Answer from the drawing. Dimensions are ordinates in mm from the lowest x, y and z of the part. Round coordinates to 2 decimals unless told otherwise and drop trailing zeros. Order: outer loops, then holes, each group sorted by start corner. A loop starts at its lowest first (then second) coordinate and runs counter-clockwise, first axis right, second up. Notation, with made-up numbers: (-21.75, 23) -> (36.25, 23) arc R28 cw to (36.25, 46) -> close; hole circle Ø5 at (77, -5). An arc over 180 degrees is marked (long way). Use a Markdown table: item, result. Add a question column.
Item 1: For a pull along Z with two mould halves and no side action, classify the marked faces 1 and 2 as +Z half, -Z half, draft (parallel to the pull), parting line (faces both ways), or undercut.
Item 2: Find the intervals of material crossed by L1, parallel to X at y = 1.1, z = 78.35; L2, parallel to X at y = 2.2, z = 78.35; L3, parallel to Y at x = 28.5, z = 90.5, in increasing order. Write a range as [from, to].
Item 3: Flat-ended cylindrical pins translate along their axes: P1, Ø1.5, axis at y = 11.5, z = 92, coming from the -X side; P2, Ø2, axis at x = 66, z = 109, coming from the +Y side; P3, Ø1.5, axis at x = 98, y = 4, coming from the +Z side; P4, Ø7, axis at x = 140.85, z = 78.35, coming from the -Y side. Find the tip coordinate at first contact, or state that the pin passes through.
Item 4: A cutting plane is placed at D-D, the plane x = 15.85. Determine the outline of the cut face in (y, z).
Item 5: A cutting plane is placed at B-B, the plane x = 78.35. Determine the outline of the cut face in (y, z).
Item 6: A cutting plane is placed at A-A, the plane z = 78.35. Determine the outline of the cut face in (x, y), plus the area to 4 significant figures.
Item 7: A cutting plane is placed at C-C, the plane z = 15.85. Determine the outline of the cut face in (x, y).
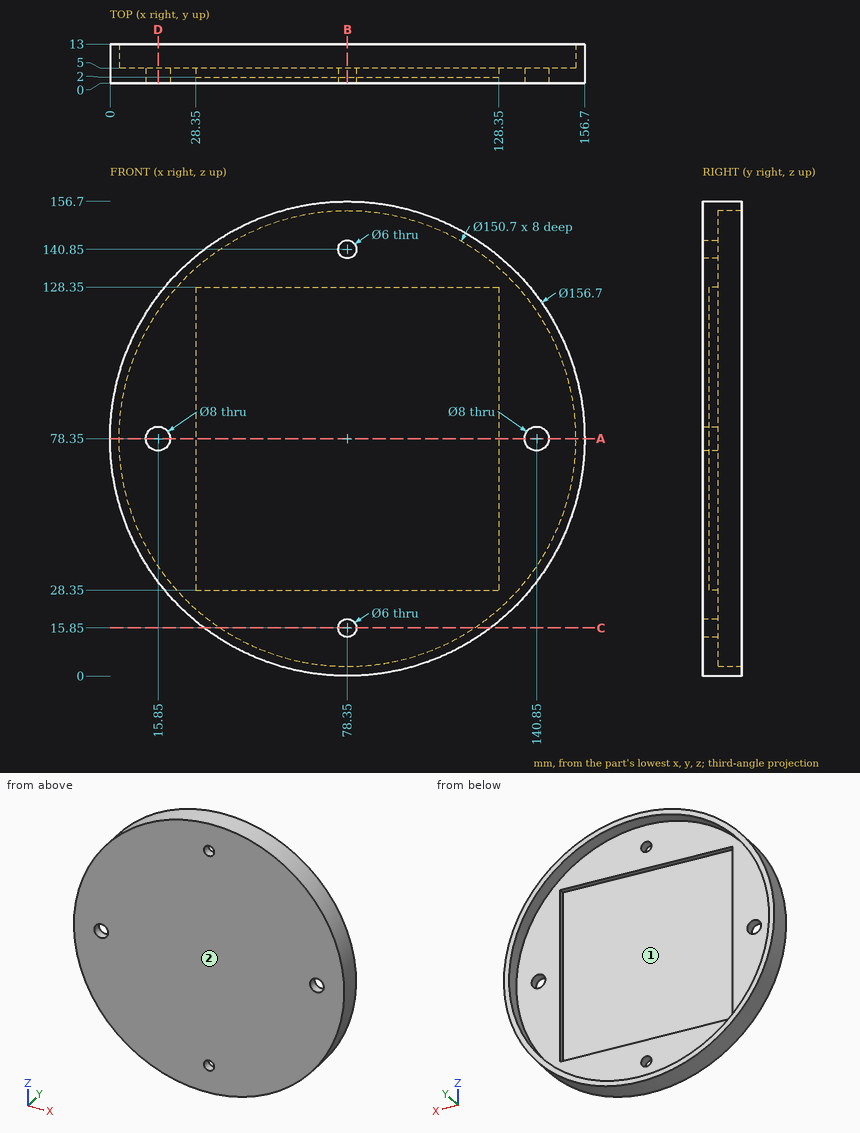
Reported:
| question | item | result |
|---|---|---|
| 1 | face 1 | undercut |
| 1 | face 2 | draft |
| 2 | L1 | [0, 11.85], [19.85, 136.85], [144.85, 156.7] |
| 2 | L2 | [0, 11.85], [19.85, 28.35], [128.35, 136.85], [144.85, 156.7] |
| 2 | L3 | [0, 2] |
| 3 | P1 | x = 1.07 |
| 3 | P2 | y = 2 |
| 3 | P3 | z = 154.39 |
| 3 | P4 | through |
| 4 | outline | (0, 31.1) -> (13, 31.1) -> (13, 36.26) -> (5, 36.26) -> (5, 74.35) -> (0, 74.35) -> close; (0, 82.35) -> (5, 82.35) -> (5, 120.44) -> (13, 120.44) -> (13, 125.6) -> (0, 125.6) -> close |
| 5 | outline | (0, 0) -> (13, 0) -> (13, 3) -> (5, 3) -> (5, 12.85) -> (0, 12.85) -> close; (0, 18.85) -> (5, 18.85) -> (5, 28.35) -> (2, 28.35) -> (2, 128.35) -> (5, 128.35) -> (5, 137.85) -> (0, 137.85) -> close; (0, 143.85) -> (5, 143.85) -> (5, 153.7) -> (13, 153.7) -> (13, 156.7) -> (0, 156.7) -> close |
| 6 | outline | (0, 0) -> (11.85, 0) -> (11.85, 5) -> (3, 5) -> (3, 13) -> (0, 13) -> close; (19.85, 0) -> (136.85, 0) -> (136.85, 5) -> (128.35, 5) -> (128.35, 2) -> (28.35, 2) -> (28.35, 5) -> (19.85, 5) -> close; (144.85, 0) -> (156.7, 0) -> (156.7, 13) -> (153.7, 13) -> (153.7, 5) -> (144.85, 5) -> close |
| 6 | area | 451.5 mm² |
| 7 | outline | (31.1, 0) -> (75.35, 0) -> (75.35, 5) -> (36.26, 5) -> (36.26, 13) -> (31.1, 13) -> close; (81.35, 0) -> (125.6, 0) -> (125.6, 13) -> (120.44, 13) -> (120.44, 5) -> (81.35, 5) -> close |
